Verification items for the finished model (mm, model axes). A direction names the side the tool comes from. Round coordinates to 2 decimals unless told otherwise and drop trailing zeros. Order: outer loops, then holes, each group sorted by start corner. A loop starts at its lowest first (then second) coordinate and runs counter-clockwise, first axis right, second up.
Autodesk Inventor part; units mm, degrees
ref_plane "YZ Plane" through (0, 0, 0) normal (1, 0, 0) x (0, 1, 0)
ref_plane "XZ Plane" through (0, 0, 0) normal (0, 1, 0) x (-1, 0, 0)
ref_plane "XY Plane" through (0, 0, 0) normal (0, 0, 1) x (1, 0, 0)
sketch "Sketch1" plane through (0, 0, 0) normal (1, 0, 0) x (0, 1, 0)
  circle A0 centre (0, 0) radius 35
  dimension "d0" = 70
extrude "Extrusion1" add sketch "Sketch1" along normal blind 5
sketch "Sketch2" plane through (5, 0, 0) normal (1, 0, 0) x (0, 0, -1)
  circle A0 centre (0, 0) radius 35
  circle A1 centre (0, 0) radius 23 construction
  point P0 (23, 0)
  point P1 (16.2635, 16.2635)
  point P2 (0, 23)
  point P3 (-16.2635, 16.2635)
  point P4 (-23, 0)
  point P5 (-16.2635, -16.2635)
  point P6 (0, -23)
  point P7 (16.2635, -16.2635)
  dimension "d3" = 46
  dimension "d6" = 360
hole "Hole1" at (5, 0, -23) at (5, 16.2635, -16.2635) at (5, 23, 0) at (5, 16.2635, 16.2635) at (5, 0, 23) at (5, -16.2635, 16.2635) at (5, -23, 0) at (5, -16.2635, -16.2635) direction (-1, 0, 0) diameter 15 end through all
sketch "Sketch3" plane through (5, 0, 0) normal (1, 0, 0) x (0, 0, -1)
  circle A0 centre (0, -23) radius 7.5
  circle A1 centre (-23, 0) radius 7.5
  circle A2 centre (0, 23) radius 7.5
  circle A3 centre (23, 0) radius 7.5
  circle A4 centre (16.2635, 16.2635) radius 7.5
  circle A5 centre (-16.2635, 16.2635) radius 7.5
  circle A6 centre (-16.2635, -16.2635) radius 7.5
  circle A7 centre (16.2635, -16.2635) radius 7.5
  circle A8 centre (0, 0) radius 35
extrude "Extrusion2" add sketch "Sketch3" along normal blind 1 contours A0 | A1 | A2 | A3 | A4 | A5 | A6 | A7 | A8
properties part number "MAGNETPLATE CONCEPT"
1) Sectioned sample at A-A on x = 2.1. Count the separate pieces of the cut face and the enclosed holes in it, then the cut area to 3 significant figures.
2) Scan lines: probe 1 along Y at (x, z) = (1.4, -2); probe 2 along Z at (x, y) = (4.2, 22); probe 3 along Y at (x, z) = (1.75, 15). Record each from-to range of solid material in increasing order.
3) Sectioned sample at D-D on y = 21. Record the cut outline in (x, z), then the cut area to 3 significant figures.
4) Draft check along Z on faces 1 (the cylindrical face through (2.465, -30.436, 0.976)), 2 (the flat face through (0, 0, 0)), 3 (the cylindrical face through (2.96, 16.51, -30.86)). Enter one of: released by +Z, released by -Z, zero draft, split by the parting line, or undercut.
5) Tool access check on faces 4 (the flat face through (5, 16, 16)), 5 (the flat face through (6, 0, 0)). Record the directions out of +Z, -Z, +X, -X, +Y, -Y that give a thin tool (end or side, any length) a straight path to the whole face; none if there is none.
6) Go/stop test with flat-tipped pins: pin 1 Ø4.5 at (y, z) = (20.5, 3) entering from -X; pin 2 Ø3 at (x, z) = (5, 2) entering from +Y; pin 3 Ø2 at (x, z) = (1.5, 9) entering from +Y. Record where each tip stops, or that it passes through.
7) Sectioned sample at B-B on y = 0. Record the cut outline in (x, z), then the cut area to 3 significant figures.
Returned:
1. separate pieces: 1
1. enclosed holes: 8
1. area: 2,430 mm2
2. probe 1: y = -34.94 to -30.23, -15.77 to 15.77, 30.23 to 34.94
2. probe 2: z = -27.22 to -21.09, -11.43 to -7.43, 7.43 to 11.43, 21.09 to 27.22
2. probe 3: y = -31.62 to -23.66, -8.87 to 8.87, 23.66 to 31.62
3. outline: (0, -28) - (6, -28) - (6, 28) - (0, 28) - (0, 22.08) - (5, 22.08) - (5, 10.45) - (0, 10.45) - (0, 7.23) - (5, 7.23) - (5, -7.23) - (0, -7.23) - (0, -10.45) - (5, -10.45) - (5, -22.08) - (0, -22.08) - close
3. area: 147 mm2
4. face 1: undercut
4. face 2: zero draft
4. face 3: split by the parting line
5. face 4: -X
5. face 5: +Z, -Z, +X, +Y, -Y
6. pin 1: stops at x = 5
6. pin 2: stops at y = 35
6. pin 3: stops at y = 34.07
7. outline: (0, -35) - (6, -35) - (6, 35) - (0, 35) - (0, 30.5) - (5, 30.5) - (5, 15.5) - (0, 15.5) - (0, -15.5) - (5, -15.5) - (5, -30.5) - (0, -30.5) - close
7. area: 270 mm2
